Autodesk Inventor part; units mm, degrees
ref_plane "YZ Plane" through (0, 0, 0) normal (1, 0, 0) x (0, 1, 0)
ref_plane "XZ Plane" through (0, 0, 0) normal (0, 1, 0) x (-1, 0, 0)
ref_plane "XY Plane" through (0, 0, 0) normal (0, 0, 1) x (1, 0, 0)
sketch "Sketch1" plane through (0, 0, 0) normal (1, 0, 0) x (0, 1, 0)
  line L0 (0, 0) -> (25.4, 0)
  line L1 (25.4, 0) -> (25.4, -736.6)
  line L2 (25.4, -736.6) -> (0, -736.6)
  line L3 (0, -736.6) -> (0, 0)
  dimension "d0" = 25.4
  dimension "d1" = 736.6
extrude "Extrusion1" add sketch "Sketch1" along normal blind 25.4
sketch "Sketch2" plane through (0, 0, 0) normal (0, 0, 1) x (1, 0, 0)
  line L0 (3.175, 3.175) -> (22.225, 3.175)
  line L1 (22.225, 3.175) -> (22.225, 22.225)
  line L2 (22.225, 22.225) -> (3.175, 22.225)
  line L3 (3.175, 22.225) -> (3.175, 3.175)
  line L4 (0, 25.4) -> (25.4, 25.4)
  line L5 (0, 0) -> (0, 25.4)
  dimension "d4" = 3.175
  dimension "d5" = 3.175
  dimension "d6" = 19.05
  dimension "d7" = 19.05
extrude "Extrusion2" cut sketch "Sketch2" against normal blind 165.1
sketch "Sketch3" plane through (0, 25.4, 0) normal (0, 1, 0) x (1, 0, 0)
  line L0 (0, 0) -> (0, 736.6)
  line L1 (0, 0) -> (12.7, 0)
  line L2 (0, 0) -> (25.4, 0)
  line L3 (12.7, 0) -> (12.7, 152.4)
  line L4 (22.225, 152.4) -> (3.175, 152.4)
  line L5 (12.7, 152.4) -> (12.7, 139.7)
  line L6 (12.7, 0) -> (12.7, 12.7)
  circle A0 centre (12.7, 12.7) radius 2.54
  circle A1 centre (12.7, 139.7) radius 2.54
  dimension "d10" = 152.4
  dimension "d11" = 12.7
  dimension "d12" = 12.7
  dimension "d13" = 5.08
extrude "Extrusion3" cut sketch "Sketch3" against normal blind 25.4
sketch "Sketch4" plane through (0, 25.4, 0) normal (0, 1, 0) x (1, 0, 0)
  line L0 (0, 736.6) -> (25.4, 736.6)
  line L1 (12.7, 736.6) -> (0, 736.6)
  line L2 (12.7, 736.6) -> (12.7, 723.9)
  line L3 (12.7, 723.9) -> (12.7, 571.5)
  line L4 (12.7, 571.5) -> (12.7, 584.2)
  circle A0 centre (12.7, 584.2) radius 2.54
  circle A1 centre (12.7, 723.9) radius 2.54
  point P0 (0, 0)
  dimension "d16" = 12.7
  dimension "d17" = 12.7
  dimension "d18" = 152.4
  dimension "d19" = 12.7
  dimension "d20" = 5.08
extrude "Extrusion4" cut sketch "Sketch4" against normal blind 25.4
properties part number "1by1by6" material "Aluminum 6061"
Source: CAD feature listing. Evaluate the final solid. Frame: model axes, mm. A direction names the side the tool comes from. Coordinates: 2 decimals unless noted, no trailing zeros. Loops run counter-clockwise (first coordinate to the right, second up) from the corner with the lowest first, then second, coordinate; pieces in that order, holes last. Notation, with made-up numbers: M 42,74 L 62,74 A17 cw 62,85 Z; hole C 70.25,58.25 d1. An arc over 180 degrees is marked long. Use a Markdown table: item, result. Add a question column.
Q1. Draft query along Y for faces 3 (the flat face through (13, 3.175, -81)), 4 (the flat face through (13, 25.4, -363)), 5 (the flat face through (25.4, 13, -363)), 6 (the flat face through (3.175, 13, -81)). Return one class per face: pulls with the +Y half, pulls with the -Y half, needs draft (parallel to the pull), parting line crosses it, or undercut.
Q2. First-contact query: pin 1 (4.5 mm diameter, centred on x = 12.7, z = -12.7, fed in from +Y). Flat tip, straight axial feed; report the tip coordinate or a pass-through.
Q3. Section query B-B, the plane y = 9. Return loops of the section in (x, z) (3 decimals), and give its area (3 significant figures).
Q4. Access query for faces 1 (the flat face through (13, 13, -736.6)), 2 (the flat face through (13, 22.225, -81)). Directions: +Z, -Z, +X, -X, +Y, -Y. A direction counts if a zero-diameter tool reaches every point of the face in a straight line with its end or side. Return the directions, or none.
Q5. Section query A-A, the plane z = -107. Return loops of the section in (x, y) (3 decimals), and give its area (3 significant figures).
Q6. Material intervals for L1, parallel to Z at x = 12.7, y = 8; L2, parallel to Z at x = 12.7, y = 1.6; L3, parallel to Z at x = 13.5, y = 20, sorted ascending.
Result:
| question | item | result |
|---|---|---|
| 1 | face 3 | undercut |
| 1 | face 4 | pulls with the +Y half |
| 1 | face 5 | needs draft |
| 1 | face 6 | undercut |
| 2 | pin 1 | passes through |
| 3 | outline | M 0,-736.6 L 25.4,-736.6 L 25.4,0 L 22.225,0 L 22.225,-165.1 L 3.175,-165.1 L 3.175,0 L 0,0 Z; hole C 12.7,-723.9 d5.08; hole C 12.7,-584.2 d5.08 |
| 3 | area | 15,500 mm2 |
| 4 | face 1 | -Z, +X, -X, +Y, -Y |
| 4 | face 2 | +Z |
| 5 | outline | M 0,0 L 25.4,0 L 25.4,25.4 L 0,25.4 Z; hole M 3.175,3.175 L 22.225,3.175 L 22.225,22.225 L 3.175,22.225 Z |
| 5 | area | 282 mm2 |
| 6 | L1 | z = -736.6 to -726.44, -721.36 to -586.74, -581.66 to -165.1 |
| 6 | L2 | z = -736.6 to -726.44, -721.36 to -586.74, -581.66 to -142.24, -137.16 to -15.24, -10.16 to 0 |
| 6 | L3 | z = -736.6 to -726.31, -721.49 to -586.61, -581.79 to -165.1 |
